The listing builds one solid part. Answer for the finished solid, in the listing's coordinates (mm). A direction names the side the tool comes from. Coordinates: 2 decimals unless noted, no trailing zeros. Loops run counter-clockwise (first coordinate to the right, second up) from the corner with the lowest first, then second, coordinate; pieces in that order, holes last. Notation, with made-up numbers: M 88,-39 L 95,-39 A21 ccw 95,-35 Z; hole C 61.5,13.25 d5. An arc over 180 degrees is marked long. Return JSON: item names as keys, results as strings. Group by question number.
1. Section B-B (z = -12.7) is taken. Write down the section's boundary in (x, y).
2. Straight lines are drawn through the part: L1, parallel to Y at x = 18.25, z = -12.7; L2, parallel to Z at x = 16.25, y = 30.5; L3, parallel to X at y = 31, z = -11. For each, find the intervals that lie inside material, in ascending order. Write a range as from..to.
3. Given P1, Ø5, axis at x = 8.5, y = 8.5, coming from the -Z side; P2, Ø12, axis at y = 28.5, z = -17, coming from the -X side; P3, Ø6, axis at y = 25.5, z = -22, coming from the +X side, each flat-ended and moving along its own axis, determine where each tip first touches the part or whether it passes through.
4. Section D-D (y = 11.5) is taken. Write down the section's boundary in (x, z), then the cut area to 3 significant figures.
5. Section A-A (y = 21.59) is taken. Write down the section's boundary in (x, z), then the cut area to 3 significant figures.
6. Which of the six approach directions +Z, -Z, +X, -X, +Y, -Y give full straight-line access (tool end or side, diameter ignored) to faces 1 (the face through (2.28, 17.69, -2.29)), 2 (the face through (23.11, 17.69, -23.12)), 3 (the face through (13, 18, -1.778))?
7. Section C-C (x = 3.5) is taken. Write down the section's boundary in (y, z), then the cut area to 3 significant figures.
```python
from build123d import *

# Parameters (mm, degrees)
SKETCH1_W           = 25.4
SKETCH1_H           = 25.4
BOSS_EXTRUDE1_DEPTH = 2.54
SKETCH2_W           = 21.844
SKETCH2_H           = 21.844
BOSS_EXTRUDE2_DEPTH = 31.75
SKETCH3_R           = 6.731
CUT_EXTRUDE1_DEPTH  = 49.774614135
CHAMFER1_SIZE       = 1.016


with BuildPart() as part:
    # Sketch1 → Boss-Extrude1 (new body)
    with BuildSketch(Plane(origin=(0, 0, 0), x_dir=(1, 0, 0), z_dir=(0, 1, 0))):
        with Locations((12.7, 12.7)):
            Rectangle(SKETCH1_W, SKETCH1_H)
    extrude(amount=BOSS_EXTRUDE1_DEPTH)

    # Sketch2 → Boss-Extrude2 (add)
    with BuildSketch(Plane(origin=(0, 2.54, 0), x_dir=(1, 0, 0), z_dir=(0, 1, 0))):
        with Locations((12.7, 12.7)):
            Rectangle(SKETCH2_W, SKETCH2_H)
    extrude(amount=BOSS_EXTRUDE2_DEPTH)

    # Sketch3 → Cut-Extrude1 (cut, through all)
    with BuildSketch(Plane.ZY.offset(-1.778)):
        with Locations((-12.7, 21.59)):
            Circle(SKETCH3_R)
    extrude(amount=-CUT_EXTRUDE1_DEPTH, mode=Mode.SUBTRACT)

    # Chamfer1
    chamfer1_edges = [part.edges().sort_by_distance(p)[0] for p in [
        (1.778, 18.415, -23.622),
        (1.778, 18.415, -1.778),
        (23.622, 18.415, -1.778),
        (23.622, 18.415, -23.622),
        (1.778, 34.29, -12.7),
        (12.7, 34.29, -1.778),
        (23.622, 34.29, -12.7),
        (12.7, 34.29, -23.622),
        (23.622, 21.59, -19.431),
        (1.778, 21.59, -19.431),
        (12.7, 0, -25.4),
        (25.4, 0, -12.7),
        (12.7, 0, 0),
        (0, 0, -12.7),
        (0, 1.27, -25.4),
        (25.4, 1.27, -25.4),
        (25.4, 1.27, 0),
        (0, 1.27, 0),
    ]]
    chamfer(chamfer1_edges, length=CHAMFER1_SIZE)


solid = part.part
```
Worked out:
{
 "1": {"outline": "M 0,1.02 L 1.02,0 L 24.38,0 L 25.4,1.02 L 25.4,2.54 L 23.62,2.54 L 23.62,13.84 L 22.61,14.86 L 2.79,14.86 L 1.78,13.84 L 1.78,2.54 L 0,2.54 Z; M 1.78,29.34 L 2.79,28.32 L 22.61,28.32 L 23.62,29.34 L 23.62,33.27 L 22.61,34.29 L 2.79,34.29 L 1.78,33.27 Z"},
 "2": {"L1": "0..14.86, 28.32..34.29", "L2": "-23.62..-1.78", "L3": "1.78..23.62"},
 "3": {"P1": "z = -23.62", "P2": "x = 1.78", "P3": "x = 23.62"},
 "4": {"outline": "M 1.78,-22.61 L 2.79,-23.62 L 22.61,-23.62 L 23.62,-22.61 L 23.62,-2.79 L 22.61,-1.78 L 2.79,-1.78 L 1.78,-2.79 Z", "area": "475 mm^2"},
 "5": {"outline": "M 1.78,-22.61 L 2.79,-23.62 L 22.61,-23.62 L 23.62,-22.61 L 23.62,-20.45 L 22.61,-19.43 L 2.79,-19.43 L 1.78,-20.45 Z; M 1.78,-4.95 L 2.79,-5.97 L 22.61,-5.97 L 23.62,-4.95 L 23.62,-2.79 L 22.61,-1.78 L 2.79,-1.78 L 1.78,-2.79 Z", "area": "179 mm^2"},
 "6": {"face 1": "+Z, -X, +Y", "face 2": "-Z, +X, +Y", "face 3": "+Z, +X, -X, +Y"},
 "7": {"outline": "M 0,-24.38 L 1.02,-25.4 L 2.54,-25.4 L 2.54,-23.62 L 33.27,-23.62 L 34.29,-22.61 L 34.29,-2.79 L 33.27,-1.78 L 2.54,-1.78 L 2.54,0 L 1.02,0 L 0,-1.02 Z; hole C 21.59,-12.7 d13.46", "area": "614 mm^2"}
}
